Can you work these out from the model? Positions are in its coordinate system, mm. A direction names the side the tool comes from. Coordinates: 2 decimals unless noted, no trailing zeros. Order: outer loops, then holes, each group sorted by start corner. A loop starts at its lowest first (then second) coordinate and runs counter-clockwise, first axis right, second up. Notation, with made-up numbers: (38, 38) -> (62, 38) arc R23 cw to (62, 74) -> close; hole circle Ø11 at (-19.75, -17.5). An arc over 180 degrees is marked (long way). Answer as CSV lines item,"result".
from build123d import *

# Parameters (mm, degrees)
SKETCH_2_R          = 6
SKETCH_2_R_2        = 4.5
CUT_EXTRUDE_1_DEPTH = 0.1
SKETCH_3_R          = 6
SKETCH_3_R_2        = 4.5
CUT_EXTRUDE_2_DEPTH = 0.1


with BuildPart() as part:
    # 草图1 → 旋转1 (revolve)
    with BuildSketch(Plane.XY, mode=Mode.PRIVATE) as revolve_1_sk:
        Polygon((3.5, 0), (3.5, 5), (8, 5), (8, 3.8), (7, 3.8), (7, 0), align=None)
    revolve(revolve_1_sk.sketch.rotate(Axis((0, 0, 0), (0, 1, 0)), 90), axis=Axis((0, 0, 0), (0, 1, 0)))

    # 草图2 → 切除-拉伸1 (cut, symmetric)
    with BuildSketch(Plane.XZ):
        with Locations(Location((0, 0, 0), (0, 0, 270))):
            Circle(SKETCH_2_R)
        with Locations(Location((0, 0, 0), (0, 0, 270))):
            Circle(SKETCH_2_R_2, mode=Mode.SUBTRACT)
    extrude(amount=CUT_EXTRUDE_1_DEPTH, both=True, mode=Mode.SUBTRACT)

    # 草图3 → 切除-拉伸2 (cut, symmetric)
    with BuildSketch(Plane(origin=(0, 5, 0), x_dir=(1, 0, 0), z_dir=(0, 1, 0))):
        with Locations(Location((0, 0, 0), (0, 0, 90))):
            Circle(SKETCH_3_R)
        with Locations(Location((0, 0, 0), (0, 0, 90))):
            Circle(SKETCH_3_R_2, mode=Mode.SUBTRACT)
    extrude(amount=CUT_EXTRUDE_2_DEPTH, both=True, mode=Mode.SUBTRACT)


solid = part.part
Q1. Imagine slicing it at C-C (x = -6.5). List the corners of the cut face in (y, z) for me, and give its area (3 significant figures).
Solution:
outline,"(0, -2.6) -> (3.8, -2.6) -> (3.8, -4.66) -> (5, -4.66) -> (5, 4.66) -> (3.8, 4.66) -> (3.8, 2.6) -> (0, 2.6) -> close"
area,"30.9 mm2"
Q2. If I drill on line 1 (X direction, y = 3, z = 0); line 2 (Y direction, x = 0.5, z = 5.25); line 3 (Y direction, x = -4.5, z = 5.75), over which ranges is the centre line in solid material (lowest first)?
Solution:
line 1,"-7 to -3.5, 3.5 to 7"
line 2,"0.1 to 4.9"
line 3,"3.8 to 5"
Q3. For P1, Ø2, axis at y = 1, z = -5.5, coming from the +X side; P2, Ø3, axis at x = 5.5, z = 1.5, coming from the -Y side, each with a flat end and sliding along its axis, tell me the tip position at first contact or that it passes through.
Solution:
P1,"x = 5.36"
P2,"y = 0"
Q4. Imagine slicing it at B-B (z = 0). List the corners of the cut face in (x, y) for me.
Solution:
outline,"(-8, 3.8) -> (-7, 3.8) -> (-7, 0) -> (-6, 0) -> (-6, 0.1) -> (-4.5, 0.1) -> (-4.5, 0) -> (-3.5, 0) -> (-3.5, 5) -> (-4.5, 5) -> (-4.5, 4.9) -> (-6, 4.9) -> (-6, 5) -> (-8, 5) -> close; (3.5, 0) -> (4.5, 0) -> (4.5, 0.1) -> (6, 0.1) -> (6, 0) -> (7, 0) -> (7, 3.8) -> (8, 3.8) -> (8, 5) -> (6, 5) -> (6, 4.9) -> (4.5, 4.9) -> (4.5, 5) -> (3.5, 5) -> close"
Q5. We'd pull the mould along Z, two halves only. Please class faces 3 (the cylindrical face through (3.105, 2.535, -1.615)), 4 (the cylindrical face through (7.81, 4.39, 1.73)), 5 (the flat face through (4, 0, 0)), 6 (the flat face through (-4.5, 4.9, 1.4)): pulls with the +Z half, pulls with the -Z half, needs draft (parallel to the pull), parting line crosses it, or undercut.
Solution:
face 3,"undercut"
face 4,"parting line crosses it"
face 5,"needs draft"
face 6,"undercut"
Q6. Imagine slicing it at D-D (y = 4.1). List the corners of the cut face in (x, z) for me, and give its area (3 significant figures).
Solution:
outline,"circle Ø16 at (0, 0); hole circle Ø7 at (0, 0)"
area,"163 mm2"
Q7. Imagine slicing it at A-A (x = 0). List the corners of the cut face in (y, z) for me, and give its area (3 significant figures).
Solution:
outline,"(0, -7) -> (3.8, -7) -> (3.8, -8) -> (5, -8) -> (5, -6) -> (4.9, -6) -> (4.9, -4.5) -> (5, -4.5) -> (5, -3.5) -> (0, -3.5) -> (0, -4.5) -> (0.1, -4.5) -> (0.1, -6) -> (0, -6) -> close; (0, 3.5) -> (5, 3.5) -> (5, 4.5) -> (4.9, 4.5) -> (4.9, 6) -> (5, 6) -> (5, 8) -> (3.8, 8) -> (3.8, 7) -> (0, 7) -> (0, 6) -> (0.1, 6) -> (0.1, 4.5) -> (0, 4.5) -> close"
area,"36.8 mm2"
Q8. Which directions (+Z, -Z, +X, -X, +Y, -Y) give clear straight access to the entire face, cutting with the end or side of a thin tool? Please do faces 1 (the flat face through (-6, 5, -2)), 2 (the flat face through (6, 3.8, -4)).
Solution:
face 1,"+Z, -Z, +X, -X, +Y"
face 2,"-Y"
